Source: CAD feature listing. Evaluate the final solid. Frame: model axes, mm. A direction names the side the tool comes from. Coordinates: 2 decimals unless noted, no trailing zeros. Order: outer loops, then holes, each group sorted by start corner. A loop starts at its lowest first (then second) coordinate and runs counter-clockwise, first axis right, second up.
```python
from build123d import *

# Parameters (mm, degrees)
EXTRUDE_1_DEPTH = 6


with BuildPart() as part:
    # 草图1 → 凸台-拉伸1 (new body)
    with BuildSketch(Plane(origin=(0, 0, 0), x_dir=(1, 0, 0), z_dir=(0, 1, 0))):
        with BuildLine():
            Line((-30, 18.027756377), (-30, -18.027756377))
            ThreePointArc((-30, -18.027756377), (35, 0), (-30, 18.027756377))
        make_face()
        with BuildLine():
            ThreePointArc((-21.324183136, 15.733061163), (-26.784109172, 16.578947368), (-23.591969867, 12.069339576))
            ThreePointArc((-23.591969867, 12.069339576), (-26.5, 0), (-23.591969867, -12.069339576))
            ThreePointArc((-23.591969867, -12.069339576), (-26.784109172, -16.578947368), (-21.324183136, -15.733061163))
            ThreePointArc((-21.324183136, -15.733061163), (7.250324934, -25.488875777), (26.412280702, -2.154397394))
            ThreePointArc((26.412280702, -2.154397394), (31.5, 0), (26.412280702, 2.154397394))
            ThreePointArc((26.412280702, 2.154397394), (7.250324934, 25.488875777), (-21.324183136, 15.733061163))
        make_face(mode=Mode.SUBTRACT)
    extrude(amount=EXTRUDE_1_DEPTH)


solid = part.part
```
1. Ray query, line 1 (Z direction, x = -27, y = 5.15); line 2 (Z direction, x = -13, y = 4.95); line 3 (Z direction, x = 12.5, y = 0.4). Return the intervals inside material, ascending.
Findings:
line 1: z = -22.27 to -16.16, -13.84 to 13.84, 16.16 to 22.27
line 2: z = -32.5 to -23.09, 23.09 to 32.5
line 3: z = -32.69 to -23.37, 23.37 to 32.69
2. Pin query (flat end, axial travel): P1, Ø2, axis at y = 2, z = -26.5, coming from the +X side. Return the tip coordinate at first contact, or that it passes through.
Findings:
P1: stops at x = 23.97
3. Section query A-A on z = 0. Return loops of the section in (x, y).
Findings:
outline: (-30, 0) - (-26.5, 0) - (-26.5, 6) - (-30, 6) - close; (31.5, 0) - (35, 0) - (35, 6) - (31.5, 6) - close
4. Section query C-C on y = 1.85. Return loops of the section in (x, z).
Findings:
outline: (-30, -18.03) arc R35 ccw (long way) to (-30, 18.03) - close; hole (-23.59, -12.07) arc R3 ccw (long way) to (-21.32, -15.73) arc R26.5 ccw to (26.41, -2.15) arc R3 ccw (long way) to (26.41, 2.15) arc R26.5 ccw to (-21.32, 15.73) arc R3 ccw (long way) to (-23.59, 12.07) arc R26.5 ccw to start
5. Access query for faces 1 (the face through (7.682, 2.958, -25.362)), 2 (the face through (17, 6, -21)). Directions: +Z, -Z, +X, -X, +Y, -Y. A direction counts if a zero-diameter tool reaches every point of the face in a straight line with its end or side. Return the directions, or none.
Findings:
face 1: +Y, -Y
face 2: +Z, -Z, +X, -X, +Y
6. Section query D-D on z = -16.5. Return loops of the section in (x, y).
Findings:
outline: (-30, 0) - (-26.83, 0) - (-26.83, 6) - (-30, 6) - close; (-21.64, 0) - (-20.74, 0) - (-20.74, 6) - (-21.64, 6) - close; (20.74, 0) - (30.87, 0) - (30.87, 6) - (20.74, 6) - close
7. Section query B-B on x = 24. Return loops of the section in (y, z), plus the area to 3 significant figures.
Findings:
outline: (0, -25.48) - (6, -25.48) - (6, -11.24) - (0, -11.24) - close; (0, 11.24) - (6, 11.24) - (6, 25.48) - (0, 25.48) - close
area: 171 mm2
8. Draft query along Z for faces 3 (the face through (17, 0, -21)), 4 (the face through (34.977, 2.958, 1.274)), 5 (the face through (31.5, 3, 0.1)). Return one class per face: released by +Z, released by -Z, zero draft, split by the parting line, or undercut.
Findings:
face 3: zero draft
face 4: split by the parting line
face 5: undercut
